from build123d import *

# Parameters (mm, degrees)
EXTRUDE_1_DEPTH     = 100
CUT_EXTRUDE_1_DEPTH = 207.155281281
FILLET_1_RADIUS     = 50
FILLET_1_LENGTH     = 10
FILLET_2_RADIUS     = 50
FILLET_2_LENGTH     = 10
SKETCH_3_R          = 40
CUT_EXTRUDE_2_DEPTH = 207.155281281


with BuildPart() as part:
    # 草圖1 → 填料-伸長1 (new body)
    with BuildSketch(Plane(origin=(0, 0, 0), x_dir=(0, 0, -1), z_dir=(1, 0, 0))):
        with BuildLine():
            Line((0, 0), (100, 0))
            ThreePointArc((100, 0), (150, 50), (100, 100))
            Line((100, 100), (0, 100))
            Line((0, 100), (0, 0))
        make_face()
    extrude(amount=EXTRUDE_1_DEPTH)

    # 草圖2 → 除料-伸長1 (cut, through all)
    with BuildSketch(Plane(origin=(100, 0, 0), x_dir=(0, 0, -1), z_dir=(1, 0, 0))):
        with BuildLine():
            Line((-26.438322174, 10), (-26.438322174, 90))
            Line((-26.438322174, 90), (100, 90))
            ThreePointArc((100, 90), (140, 50), (100, 10))
            Line((100, 10), (-26.438322174, 10))
        make_face()
    extrude(amount=-CUT_EXTRUDE_1_DEPTH, mode=Mode.SUBTRACT)

    # 圓角1: full round fillet: the end face becomes a half cylinder, R = half its width
    fillet_1_face = Plane((50, 95, 0), x_dir=(0, 1, 0), z_dir=(0, 0, 1))  # on the end face: x along it, z out of the body
    fillet_1_slab = fillet_1_face.offset(-FILLET_1_RADIUS / 2) * Box(FILLET_1_LENGTH, 2 * FILLET_1_RADIUS, FILLET_1_RADIUS, mode=Mode.PRIVATE)  # the body's end, R deep
    fillet_1_round = Plane((50, 95, -50), x_dir=(0, 0, 1), z_dir=(0, 1, 0)) * Cylinder(FILLET_1_RADIUS, FILLET_1_LENGTH, mode=Mode.PRIVATE)  # its axis R under the face
    add(fillet_1_slab - fillet_1_round, mode=Mode.SUBTRACT)

    # 圓角2: full round fillet: the end face becomes a half cylinder, R = half its width
    fillet_2_face = Plane((50, 5, 0), x_dir=(0, -1, 0), z_dir=(0, 0, 1))  # on the end face: x along it, z out of the body
    fillet_2_slab = fillet_2_face.offset(-FILLET_2_RADIUS / 2) * Box(FILLET_2_LENGTH, 2 * FILLET_2_RADIUS, FILLET_2_RADIUS, mode=Mode.PRIVATE)  # the body's end, R deep
    fillet_2_round = Plane((50, 5, -50), x_dir=(0, 0, 1), z_dir=(0, -1, 0)) * Cylinder(FILLET_2_RADIUS, FILLET_2_LENGTH, mode=Mode.PRIVATE)  # its axis R under the face
    add(fillet_2_slab - fillet_2_round, mode=Mode.SUBTRACT)

    # 草圖3 → 除料-伸長2 (cut, through all)
    with BuildSketch(Plane(origin=(0, 100, 0), x_dir=(1, 0, 0), z_dir=(0, 1, 0))):
        with Locations(Location((50, 50, 0), (0, 0, 270))):
            Circle(SKETCH_3_R)
    extrude(amount=-CUT_EXTRUDE_2_DEPTH, mode=Mode.SUBTRACT)


solid = part.part
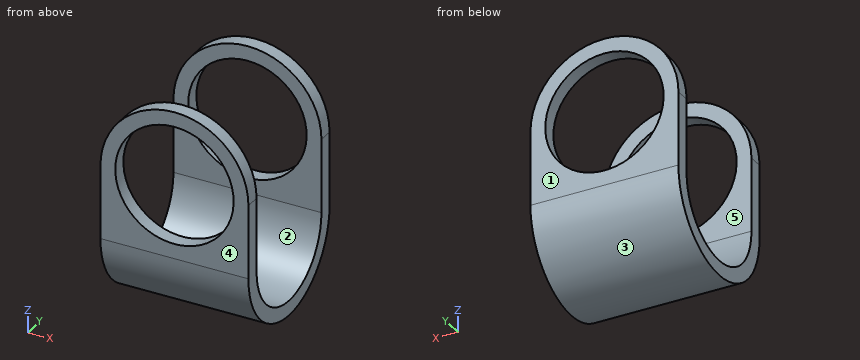
Geometry: final body of the model. Coordinates: model frame, mm. Face numbers are marked on the shaded views. A direction names the side the tool comes from. Give positions to 0.01 mm unless a question says otherwise; leave off trailing zeros. Loops run counter-clockwise (first coordinate to the right, second up) from the corner with the lowest first, then second, coordinate; pieces in that order, holes last. Notation, with made-up numbers: (76.25, 80) - (119.25, 80) arc R15 ccw to (119.25, 104) - close; hole circle Ø7 at (52.25, -25.5). An arc over 180 degrees is marked (long way). One line per question, with ' | ' between items. Start each with the question number.
(1) Section query D-D on x = 88. Return loops of the section in (y, z), then the cut area to 3 significant figures.
(2) Ray query, line 1 (X direction, y = 94.25, z = -50); line 2 (Y direction, x = 96, z = -117.5). Return the intervals inside material, ascending. Write a range as from..to.
(3) Section query A-A on x = 50. Return loops of the section in (y, z).
(4) Reachability of the marked faces 4 and 5 from +Z, -Z, +X, -X, +Y, -Y: full face, straight path, thin tool, end or side. Return the list, or none.
(5) Contact query for flat-ended pins moving along their axis: pin 1 (8 mm diameter, centred on x = 11, z = -44, fed in from +Y); pin 2 (3 mm diameter, centred on x = 77, y = 55.5, fed in from -Z); pin 3 (1.5 mm diameter, centred on x = 13.5, y = 44, fed in from -Z); pin 4 (10 mm diameter, centred on x = 42, y = 57, fed in from +Z). Output: stop coordinate, or through.
(6) Pull-direction query (Y, two-part tool) for the marked faces 1, 2 and 3; classes: released by +Y, released by -Y, zero draft, split by the parting line, or undercut.
(7) Section query B-B on z = -43. Return loops of the section in (x, y), then the cut area to 3 significant figures.
(8) Section query C-C on z = -137.5. Return loops of the section in (x, y).
The answers:
1) outline: (0, -100) arc R50 ccw to (100, -100) - (100, -62.49) - (90, -62.49) - (90, -100) arc R40 cw to (10, -100) - (10, -62.49) - (0, -62.49) - close; (0, -37.51) - (10, -37.51) - (10, -17.5) - (0, -17.5) - close; (90, -37.51) - (100, -37.51) - (100, -17.5) - (90, -17.5) - close | area: 2,560 mm2
2) line 1: 0..10, 90..100 | line 2: 3.16..14.03, 85.97..96.84
3) outline: (0, -100) arc R50 ccw to (100, -100) - (100, -90) - (90, -90) - (90, -100) arc R40 cw to (10, -100) - (10, -90) - (0, -90) - close; (0, -10) - (10, -10) - (10, 0) - (0, 0) - close; (90, -10) - (100, -10) - (100, 0) - (90, 0) - close
4) face 4: +Z, -Z, +X, -X, -Y | face 5: +Z, +X, -X
5) pin 1: y = 100 | pin 2: z = -149.84 | pin 3: z = -149.72 | pin 4: z = -138.16
6) face 1: released by +Y | face 2: undercut | face 3: split by the parting line
7) outline: (0.49, 0) - (10.62, 0) - (10.62, 10) - (0.49, 10) - close; (0.49, 90) - (10.62, 90) - (10.62, 100) - (0.49, 100) - close; (89.38, 0) - (99.51, 0) - (99.51, 10) - (89.38, 10) - close; (89.38, 90) - (99.51, 90) - (99.51, 100) - (89.38, 100) - close | area: 405 mm2
8) outline: (0, 16.93) - (100, 16.93) - (100, 36.08) - (0, 36.08) - close; (0, 63.92) - (100, 63.92) - (100, 83.07) - (0, 83.07) - close
